from build123d import *

# Parameters (mm, degrees)
CROQUIS1_R                 = 5
SALIENTE_EXTRUIR1_DEPTH    = 4
CROQUIS2_R                 = 3.35
SALIENTE_EXTRUIR2_DEPTH    = 32
CORTAR_EXTRUIR1_DEPTH      = 1.3
CORTAR_EXTRUIR1_DEPTH_BACK = 2.5


with BuildPart() as part:
    # Croquis1 → Saliente-Extruir1 (new body)
    with BuildSketch(Plane(origin=(0, 0, 0), x_dir=(1, 0, 0), z_dir=(0, 1, 0))):
        Circle(CROQUIS1_R)
    extrude(amount=SALIENTE_EXTRUIR1_DEPTH)

    # Croquis2 → Saliente-Extruir2 (add)
    with BuildSketch(Plane(origin=(0, 0, 0), x_dir=(1, 0, 0), z_dir=(0, 1, 0))):
        Circle(CROQUIS2_R)
    extrude(amount=-SALIENTE_EXTRUIR2_DEPTH)

    # Croquis4 → Cortar-Extruir1 (cut, two sides)
    with BuildSketch(Plane(origin=(0, 3.7, 0), x_dir=(1, 0, 0), z_dir=(0, 1, 0))) as cortar_extruir1_sk:
        Polygon((3.75277675, 0), (1.876388375, 3.25), (-1.876388375, 3.25), (-3.75277675, 0), (-1.876388375, -3.25), (1.876388375, -3.25), align=None)
    extrude(amount=CORTAR_EXTRUIR1_DEPTH, mode=Mode.SUBTRACT)
    extrude(cortar_extruir1_sk.sketch, amount=-CORTAR_EXTRUIR1_DEPTH_BACK, mode=Mode.SUBTRACT)


solid = part.part
Check sheet for the modelled part. Datum: model origin and axes. Units: mm. A direction names the side the tool comes from. Give positions to 0.01 mm unless a question says otherwise; leave off trailing zeros. Order: outer loops, then holes, each group sorted by start corner. A loop starts at its lowest first (then second) coordinate and runs counter-clockwise, first axis right, second up. Notation, with made-up numbers: (78.5, -12) - (131.5, -12) arc R25 ccw to (131.5, 8) - close; hole circle Ø10 at (38.25, 20.25). An arc over 180 degrees is marked (long way). Answer as CSV lines item,"result".
1. Section check A-A (x = 0). Record the boundary of the cut face in (y, z).
Result sheet:
outline,"(-32, -3.35) - (0, -3.35) - (0, -5) - (4, -5) - (4, -3.25) - (1.2, -3.25) - (1.2, 3.25) - (4, 3.25) - (4, 5) - (0, 5) - (0, 3.35) - (-32, 3.35) - close"
2. Mould release check, pull along X, two halves, no side actions. Record for faces 3 (the face through (-3.347, -15.776, -0.147)), 4 (the face through (0, 3, -3.25)), 5 (the face through (-1.2, 0, 3.3)): released by +X, released by -X, zero draft, split by the parting line, or undercut.
Result sheet:
face 3,"split by the parting line"
face 4,"undercut"
face 5,"zero draft"
3. Section check C-C (y = -7.5). Record the boundary of the cut face in (x, z), then the cut area to 3 significant figures.
Result sheet:
outline,"circle Ø6.7 at (0, 0)"
area,"35.3 mm²"
4. Scan lines: probe 1 along Y at (x, z) = (3.5, 3.5); probe 2 along Y at (x, z) = (-3, 1); probe 3 along X at (y, z) = (-11.5, -2.25). Record each from-to range of solid material in increasing order. Write a range as from..to.
Result sheet:
probe 1,"0..4"
probe 2,"-32..1.2"
probe 3,"-2.48..2.48"
5. Tool access check on faces 1 (the face through (-2.83, 2.58, 1.6)), 2 (the face through (0, -32, 0)). Record the directions out of +Z, -Z, +X, -X, +Y, -Y that give a thin tool (end or side, any length) a straight path to the whole face; none if there is none.
Result sheet:
face 1,"+Y"
face 2,"+Z, -Z, +X, -X, -Y"
6. Go/stop test with flat-tipped pins: P1, Ø3, axis at x = 1.5, y = -23, coming from the +Z side; P2, Ø5, axis at x = -0.5, z = -0.5, coming from the +Y side; P3, Ø4, axis at y = -24, z = -2.5, coming from the -X side. Record where each tip stops, or that it passes through.
Result sheet:
P1,"z = 3.35"
P2,"y = 1.2"
P3,"x = -3.31"
7. Section check D-D (z = 4). Record the boundary of the cut face in (x, y), then the cut area to 3 significant figures.
Result sheet:
outline,"(-3, 0) - (3, 0) - (3, 4) - (-3, 4) - close"
area,"24.0 mm²"
8. Section check B-B (z = 0.75). Record the boundary of the cut face in (x, y).
Result sheet:
outline,"(-4.94, 0) - (-3.26, 0) - (-3.26, -32) - (3.26, -32) - (3.26, 0) - (4.94, 0) - (4.94, 4) - (3.32, 4) - (3.32, 1.2) - (-3.32, 1.2) - (-3.32, 4) - (-4.94, 4) - close"
